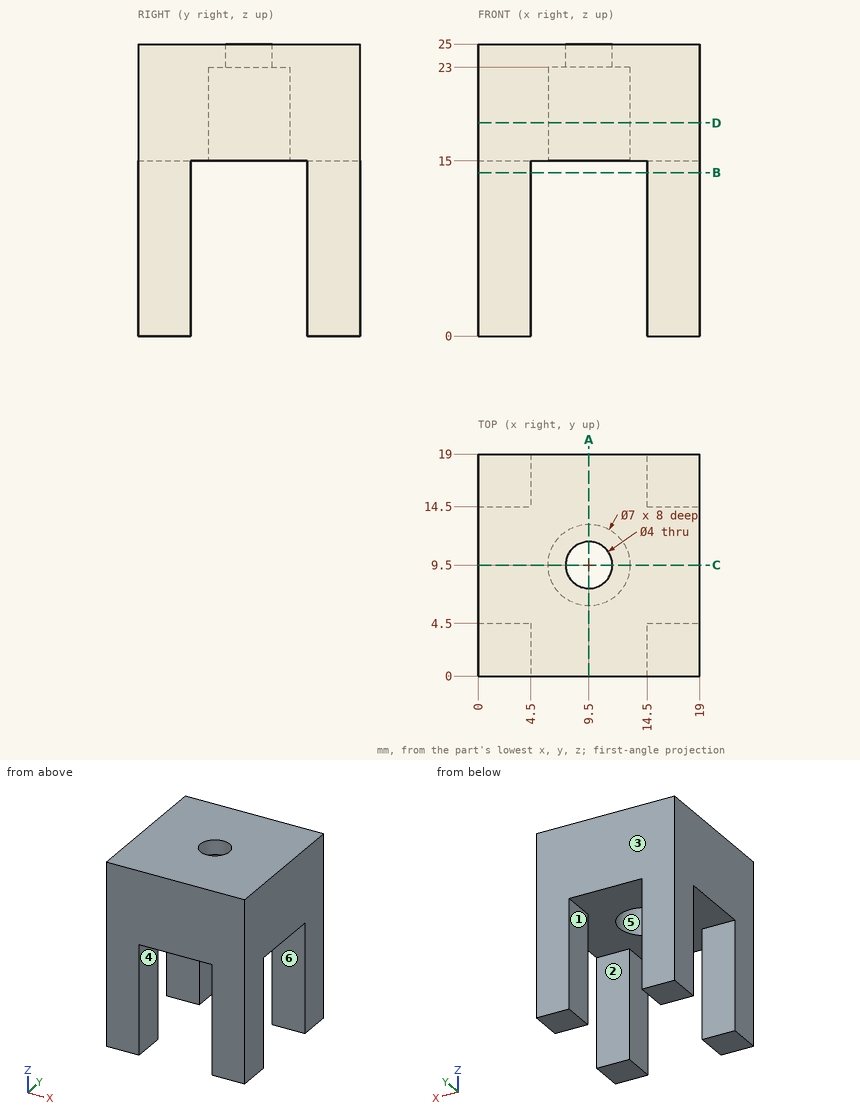
Here's the drawing with two shaded views (mm, measured from the low corner). I have some questions. A direction names the side the tool comes from. Coordinates: 2 decimals unless noted, no trailing zeros. Loops run counter-clockwise (first coordinate to the right, second up) from the corner with the lowest first, then second, coordinate; pieces in that order, holes last. Notation, with made-up numbers: M 3.5,-27.75 L 45.5,-27.75 A34 cw 45.5,4.25 Z; hole C -6,51.5 d6. An arc over 180 degrees is marked long. Put each result on its own line as item: value. Start each with the question number.
(1) Which directions (+Z, -Z, +X, -X, +Y, -Y) give clear straight access to the entire face, cutting with the end or side of a thin tool? Please do the marked faces 4, 5 and 6.
(2) We'd pull the mould along Y, two halves only. Please class the marked faces 1, 2 and 3: +Y half, -Y half, draft (parallel to the pull), parting line (faces both ways), or undercut.
(3) Imagine slicing it at A-A on x = 9.5. List the corners of the cut face in (y, z) for me.
(4) Will these pins go through, and if not, where does the flat tip stop? pin 1 Ø5 at (y, z) = (2, 8) entering from -X; pin 2 Ø5.5 at (x, y) = (10.5, 10) entering from -Z; pin 3 Ø6.5 at (x, y) = (9.5, 9.5) entering from -Z.
(5) I need wall thicknesses on probe 1 along X at (y, z) = (9.5, 24.05); probe 2 along X at (y, z) = (9.5, 21). Which ranges of each line are inside material? Lowest first, please.
(6) Imagine slicing it at B-B on z = 14. List the corners of the cut face in (x, y) for me, and give its area (3 significant figures).
(7) Imagine slicing it at D-D on z = 18.25. List the corners of the cut face in (x, y) for me.
Worked answers:
1. face 4: -Z, +Y, -Y
1. face 5: -Z
1. face 6: -Z, +X, -X
2. face 1: draft
2. face 2: undercut
2. face 3: +Y half
3. outline: M 0,15 L 6,15 L 6,23 L 7.5,23 L 7.5,25 L 0,25 Z; M 11.5,23 L 13,23 L 13,15 L 19,15 L 19,25 L 11.5,25 Z
4. pin 1: stops at x = 0
4. pin 2: stops at z = 15
4. pin 3: stops at z = 23
5. probe 1: x = 0 to 7.5, 11.5 to 19
5. probe 2: x = 0 to 6, 13 to 19
6. outline: M 0,0 L 4.5,0 L 4.5,4.5 L 0,4.5 Z; M 0,14.5 L 4.5,14.5 L 4.5,19 L 0,19 Z; M 14.5,0 L 19,0 L 19,4.5 L 14.5,4.5 Z; M 14.5,14.5 L 19,14.5 L 19,19 L 14.5,19 Z
6. area: 81.0 mm2
7. outline: M 0,0 L 19,0 L 19,19 L 0,19 Z; hole C 9.5,9.5 d7
